Can you work these out from the drawing? Everything is in mm from the part's minimum corner. A direction names the side the tool comes from. Give positions to 0.01 mm unless a question says otherwise; leave off trailing zeros. Write each loop counter-clockwise with the first axis right and the second up, starting at its lowest first coordinate (ties: lowest second). Pieces come first, ordered by that corner, then holes. Notation, with made-up numbers: (3, -8) - (12, -8) arc R32 cw to (12, 22) - close; hole circle Ø10 at (86.25, -29). An arc over 180 degrees is marked (long way). Return JSON: item names as keys, results as strings. Group by question number.
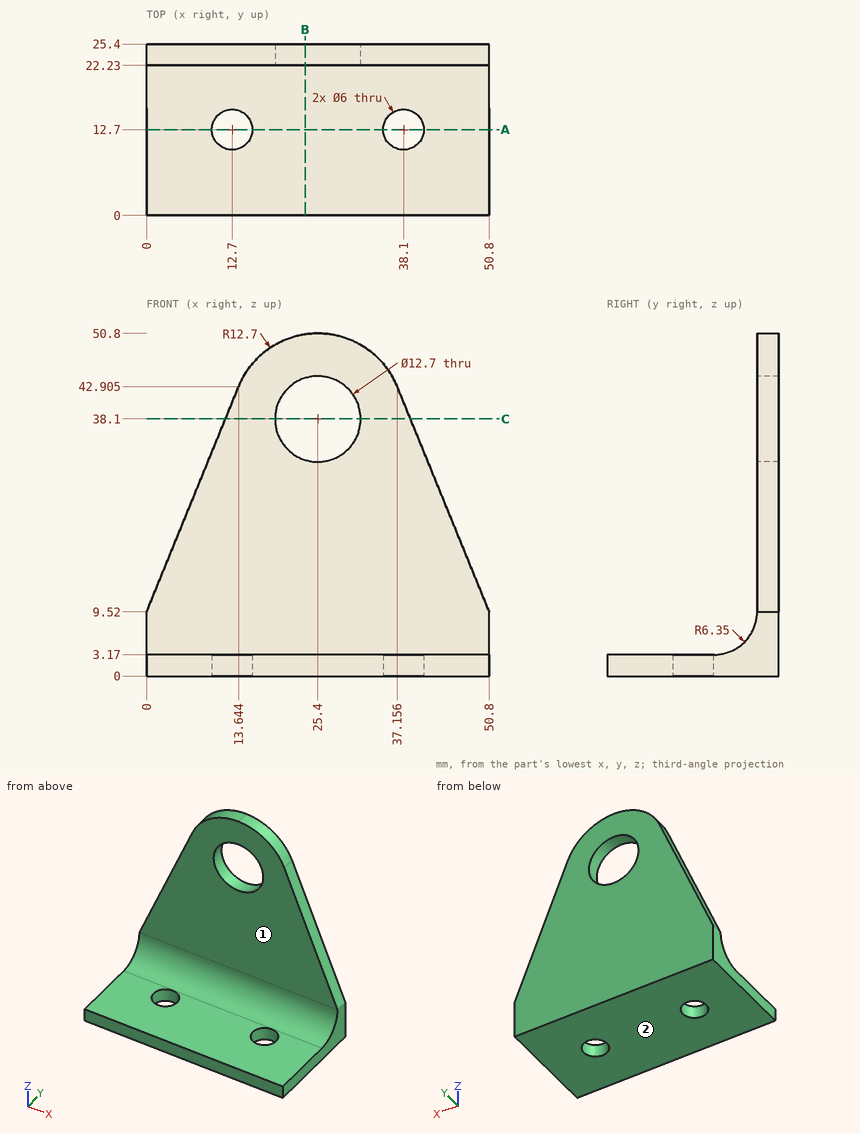
1) On a 3-axis mill with a long thin cutter (end or side, diameter ignored), from which of +Z, -Z, +X, -X, +Y, -Y can I reach the whole of each face in a straight line? I mean the marked faces 1 and 2. Say none if no direction works.
2) I need wall thicknesses on line 1 along Z through (x, y) = (25.4, 23); line 2 along Y through (x, z) = (12.7, 1.8); line 3 along Y through (x, z) = (18, 17.5). Which ranges of each line are inside material? Lowest first, please.
3) Imagine slicing it at A-A, the plane y = 12.7. Write out the boundary of the cut face in (x, z), and give its area (3 significant figures).
4) Imagine slicing it at B-B, the plane x = 23.5. Write out the boundary of the cut face in (y, z).
5) Imagine slicing it at C-C, the plane z = 38.1. Write out the boundary of the cut face in (x, y).
6) Will these pins go through, and if not, where does the flat tip stop? pin 1 Ø8 at (x, y) = (33, 10) entering from +Z; pin 2 Ø8 at (y, z) = (21, 20) entering from -X; pin 3 Ø4 at (x, z) = (17, 14) entering from -Y.
Resolved:
{
 "1": {"face 1": "+Z, +X, -X, -Y", "face 2": "-Z, +X, -X, +Y, -Y"},
 "2": {"line 1": "0 to 31.75, 44.45 to 50.8", "line 2": "0 to 9.7, 15.7 to 25.4", "line 3": "22.23 to 25.4"},
 "3": {"outline": "(0, 0) - (9.7, 0) - (9.7, 3.17) - (0, 3.17) - close; (15.7, 0) - (35.1, 0) - (35.1, 3.17) - (15.7, 3.17) - close; (41.1, 0) - (50.8, 0) - (50.8, 3.17) - (41.1, 3.17) - close", "area": "123 mm^2"},
 "4": {"outline": "(0, 0) - (25.4, 0) - (25.4, 32.04) - (22.23, 32.04) - (22.23, 9.52) arc R6.35 cw to (15.88, 3.17) - (0, 3.17) - close; (22.23, 44.16) - (25.4, 44.16) - (25.4, 50.66) - (22.23, 50.66) - close"},
 "5": {"outline": "(11.68, 22.23) - (19.05, 22.23) - (19.05, 25.4) - (11.68, 25.4) - close; (31.75, 22.23) - (39.12, 22.23) - (39.12, 25.4) - (31.75, 25.4) - close"},
 "6": {"pin 1": "z = 3.17", "pin 2": "x = 2.73", "pin 3": "y = 22.23"}
}
